Could you check a few things on this model? Use its own coordinates, in mm. A direction names the side the tool comes from. Give positions to 0.01 mm unless a question says otherwise; leave off trailing zeros. Write each loop counter-clockwise with the first axis right and the second up, starting at its lowest first coordinate (ties: lowest second). Pieces come first, ordered by that corner, then holes. Notation, with made-up numbers: (-18, 2.25) - (-13, 2.25) arc R16 ccw to (-13, 27.25) - close; hole circle Ø3 at (50, -9). An arc over 180 degrees is marked (long way). Write item = value, one per line.
from build123d import *

# Parameters (mm, degrees)
SKETCH1_W           = 30
SKETCH1_H           = 15
BOSS_EXTRUDE1_DEPTH = 70
SKETCH2_R           = 2
CUT_EXTRUDE1_DEPTH  = 5
CUT_EXTRUDE2_START  = -5
SKETCH3_R           = 10
CUT_EXTRUDE2_DEPTH  = 55


with BuildPart() as part:
    # Sketch1 → Boss-Extrude1 (new body)
    with BuildSketch(Plane(origin=(0, 0, 0), x_dir=(1, 0, 0), z_dir=(0, 1, 0))):
        Rectangle(SKETCH1_W, SKETCH1_H)
    extrude(amount=BOSS_EXTRUDE1_DEPTH)

    # Sketch2 → Cut-Extrude1 (cut)
    with BuildSketch(Plane(origin=(0, 70, 0), x_dir=(1, 0, 0), z_dir=(0, 1, 0))):
        with Locations((0, -7.5)):
            Circle(SKETCH2_R)
    extrude(amount=-CUT_EXTRUDE1_DEPTH, mode=Mode.SUBTRACT)

    # Sketch3 → Cut-Extrude2 (cut)
    with BuildSketch(Plane(origin=(0, 70, 0), x_dir=(1, 0, 0), z_dir=(0, 1, 0)).offset(CUT_EXTRUDE2_START)):
        with Locations((0, -7.5)):
            Circle(SKETCH3_R)
    extrude(amount=-CUT_EXTRUDE2_DEPTH, mode=Mode.SUBTRACT)


solid = part.part
1. If we section it at B-B, the plane z = -1.5: Please give me the cut outline in (x, y).
Filled sheet:
outline = (-15, 0) - (15, 0) - (15, 70) - (-15, 70) - close; hole (-4.36, 10) - (4.36, 10) - (4.36, 65) - (-4.36, 65) - close
2. Which directions (+Z, -Z, +X, -X, +Y, -Y) give clear straight access to the entire face, cutting with the end or side of a thin tool? Please do faces 4 (the face through (0.2, 37.9, -2.5)), 5 (the face through (0, 70, 0)), 6 (the face through (0, 67.5, 5.5)).
Filled sheet:
face_4 = +Z
face_5 = +Z, -Z, +X, -X, +Y
face_6 = +Z, +Y
3. For pin 1 (1.5 mm diameter, centred on x = 0.5, y = 37.5, fed in from +Z); pin 2 (1.5 mm diameter, centred on x = 8.5, y = 39, fed in from +Z), each with a flat end and sliding along its axis, tell me the tip position at first contact or that it passes through.
Filled sheet:
pin_1 = -2.42
pin_2 = 3.7
4. Thinking about a two-plate mould opening in X: for faces 1 (the face through (0, 35, -7.5)), 2 (the face through (15, 35, 0)), 3 (the face through (0, 65, 4)), which applies, pulls with the +X half, pulls with the -X half, needs draft (parallel to the pull), parting line crosses it, or undercut?
Filled sheet:
face_1 = needs draft
face_2 = pulls with the +X half
face_3 = undercut
5. If we section it at A-A, the plane x = 0: Please give me the cut outline in (y, z), and give its area (3 significant figures).
Filled sheet:
outline = (0, -7.5) - (70, -7.5) - (70, 5.5) - (65, 5.5) - (65, -2.5) - (10, -2.5) - (10, 7.5) - (0, 7.5) - close
area = 490 mm2
6. If we section it at D-D, the plane x = -3.5: Please give me the cut outline in (y, z).
Filled sheet:
outline = (0, -7.5) - (70, -7.5) - (70, 7.5) - (65, 7.5) - (65, -1.87) - (10, -1.87) - (10, 7.5) - (0, 7.5) - close
7. I need wall thicknesses on line 1 (Y direction, x = 2, z = 2.5); line 2 (X direction, y = 14, z = 3); line 3 (X direction, y = 56.5, z = 0). Which ranges of each line are inside material? Lowest first, please.
Filled sheet:
line_1 = 0 to 10, 65 to 70
line_2 = -15 to -8.93, 8.93 to 15
line_3 = -15 to -6.61, 6.61 to 15
8. If we section it at C-C, the plane y = 14: Please give me the cut outline in (x, z).
Filled sheet:
outline = (-15, -7.5) - (15, -7.5) - (15, 7.5) - (10, 7.5) arc R10 cw to (-10, 7.5) - (-15, 7.5) - close
